Autodesk Inventor part; units mm, degrees
ref_plane "YZ Plane" through (0, 0, 0) normal (1, 0, 0) x (0, 1, 0)
ref_plane "XZ Plane" through (0, 0, 0) normal (0, 1, 0) x (-1, 0, 0)
ref_plane "XY Plane" through (0, 0, 0) normal (0, 0, 1) x (1, 0, 0)
sketch "Náčrt1" plane through (0, 0, 0) normal (0, 1, 0) x (-1, 0, 0)
  line L0 (-49.75, 49.75) -> (49.75, 49.75)
  line L1 (49.75, 49.75) -> (49.75, -49.75)
  line L2 (49.75, -49.75) -> (-49.75, -49.75)
  line L3 (-49.75, -49.75) -> (-49.75, 49.75)
  line L4 (-49.75, 49.75) -> (49.75, -49.75) construction
  line L5 (49.75, 49.75) -> (-49.75, -49.75) construction
  line L6 (-17.75, 49.75) -> (-17.75, 24)
  line L7 (-17.75, 24) -> (-49.75, 24)
  line L8 (-49.75, -24) -> (-17.75, -24)
  line L9 (-17.75, -24) -> (-17.75, -49.75)
  circle A0 centre (-22.9375, -19) radius 1.75
  circle A1 centre (-22.9375, 19) radius 1.75
  circle A2 centre (-8.75, -42.25) radius 1.75
  circle A3 centre (39.7631, -20) radius 1.75
  circle A4 centre (39.7631, 20) radius 1.75
  circle A5 centre (-8.75, 42.25) radius 1.75
  circle A6 centre (41.75, 40.6105) radius 5
  circle A7 centre (41.75, -40.6105) radius 5
  line L10 (41.75, 40.6105) -> (41.75, 49.75) construction
  line L11 (41.75, -40.6105) -> (41.75, -49.75) construction
  line L12 (39.7631, 20) -> (39.7631, 0) construction
  line L13 (39.7631, 0) -> (39.7631, -20) construction
  line L14 (-39.25, 24) -> (-39.25, -24)
  point P0 (0, 0)
  point P1 (-33.75, 24)
  dimension "d16" = 75
  dimension "d0" = 99.5
  dimension "d1" = 99.5
  dimension "d2" = 32
  dimension "d5" = 3.5
  dimension "d7" = 7.5
  dimension "d8" = 7.5
  dimension "d9" = 5
  dimension "d10" = 5
  dimension "d11" = 10.8125
  dimension "d12" = 9
  dimension "d13" = 9.9869
  dimension "d26" = 81.221
  dimension "d27" = 10
  dimension "d28" = 8
  dimension "d31" = 40
  dimension "d32" = 48
  dimension "d33" = 10.5
extrude "Vysunutí1" add sketch "Náčrt1" along normal blind 5 contours L0 L1 L2 L9 L8 L14 L7 L6 | A0 | A1 | A2 | A3 | A4 | A5
sketch "Náčrt2" plane through (-49.75, 0, 49.75) normal (0, 0, 1) x (1, 0, 0)
  line L0 (0, 0) -> (67.5, 0)
  line L1 (0, 0) -> (1.3397, 5)
  line L2 (0, 5) -> (67.5, 5)
  line L3 (0, 0) -> (0, 5)
  line L4 (0, 5) -> (0, 0)
  point P0 (49.75, 0)
  point P1 (99.5, 0)
  point P2 (99.5, 5)
  dimension "d16" = 75
extrude "Vysunutí2" cut sketch "Náčrt2" against normal through all
hole "Díra1" at (22.9375, 0, 19) at (22.9375, 0, -19) at (8.75, 0, -42.25) at (-39.7631, 0, -20) at (-39.7631, 0, 20) at (8.75, 0, 42.25) direction (0, 1, 0) diameter 3.5 end through all countersink diameter 7.5 countersink angle 90
properties part number "new_plech" material "Stainless Steel"
Source: CAD feature listing. Evaluate the final solid. Frame: model axes, mm. A direction names the side the tool comes from. Coordinates: 2 decimals unless noted, no trailing zeros. Write each loop counter-clockwise with the first axis right and the second up, starting at its lowest first coordinate (ties: lowest second). Pieces come first, ordered by that corner, then holes. Notation, with made-up numbers: (53, -31) -> (96, -31) arc R23 cw to (96, -11) -> close; hole circle Ø10 at (35.25, 57.5). An arc over 180 degrees is marked (long way). Return JSON: item names as keys, results as strings. Group by question number.
1) Ray query, line 1 along Z through (x, y) = (8.75, 2.9); line 2 along X through (y, z) = (3.55, 42.25); line 3 along X through (y, z) = (4.2, 18.5). Return the intervals inside material, ascending.
2) Section query B-B, the plane x = 33.5. Return loops of the section in (y, z).
3) Mould query, pull axis Z, two halves, no side actions, for faces 1 (the face through (28, 2, 24)), 2 (the face through (-41.594, 1.875, 20.406)), 3 (the face through (39.25, 2, 0)). Classes: +Z half, -Z half, draft (parallel to the pull), parting line (faces both ways), or undercut.
4) Set-up query: faces 4 (the face through (17.75, 2, 37)), 5 (the face through (21.2, 3.5, -18.8)), 6 (the face through (17.75, 2, -37)). Return all of +Z, -Z, +X, -X, +Y, -Y with unobstructed straight access to the full face (end or side cutting, diameter ignored); none if empty.
5) Contact query for flat-ended pins moving along their axis: P1, Ø1.5, axis at y = 2, z = -31.5, coming from the +X side; P2, Ø2, axis at y = 3, z = 9, coming from the -X side; P3, Ø1.5, axis at x = 28, y = 2, coming from the +Z side. Output: stop coordinate, or through.
6) Section query A-A, the plane y = 0.85. State how many separate pieces and enclosed holes the cut face has, plus the area to 3 significant figures.
From the geometry:
{
 "1": {"line 1": "-49.75 to -44, -40.5 to 40.5, 44 to 49.75", "line 2": "-48.8 to -46.47, -37.03 to 7, 10.5 to 17.75", "line 3": "-48.62 to -40.66, -38.86 to 21.26, 24.61 to 39.25"},
 "2": {"outline": "(0, -24) -> (5, -24) -> (5, 24) -> (0, 24) -> close"},
 "3": {"face 1": "+Z half", "face 2": "undercut", "face 3": "draft"},
 "4": {"face 4": "+Z, +X, +Y, -Y", "face 5": "+Y, -Y", "face 6": "-Z, +X, +Y, -Y"},
 "5": {"P1": "x = 17.75", "P2": "x = -49.21", "P3": "z = 24"},
 "6": {"separate pieces": "1", "enclosed holes": "8", "area": "7,410 mm²"}
}
